```python
from build123d import *

# Parameters (mm, degrees)
SKETCH1_R           = 14
SKETCH1_R_2         = 12.425
BOSS_EXTRUDE1_DEPTH = 30
SKETCH2_W           = 40
SKETCH2_H           = 3
BOSS_EXTRUDE2_DEPTH = 30
SKETCH3_R           = 1.5
CUT_EXTRUDE1_DEPTH  = 30


with BuildPart() as part:
    # Sketch1 → Boss-Extrude1 (new body)
    with BuildSketch(Plane(origin=(0, 0, 0), x_dir=(1, 0, 0), z_dir=(0, 1, 0))):
        with Locations(Location((0, 0, 0), (0, 0, 270))):
            Circle(SKETCH1_R)
        with Locations(Location((0, 0, 0), (0, 0, 270))):
            Circle(SKETCH1_R_2, mode=Mode.SUBTRACT)
    extrude(amount=BOSS_EXTRUDE1_DEPTH)

    # Sketch2 → Boss-Extrude2 (add)
    with BuildSketch(Plane.XZ):
        with Locations((0, -14)):
            Rectangle(SKETCH2_W, SKETCH2_H)
    extrude(amount=-BOSS_EXTRUDE2_DEPTH)

    # Sketch3 → Cut-Extrude1 (cut)
    with BuildSketch(Plane.XY.offset(-12.5)):
        with Locations((17, 23)):
            Circle(SKETCH3_R)
        with Locations((-17, 23)):
            Circle(SKETCH3_R)
        with Locations((17, 7)):
            Circle(SKETCH3_R)
        with Locations((-17, 7)):
            Circle(SKETCH3_R)
    extrude(amount=-CUT_EXTRUDE1_DEPTH, mode=Mode.SUBTRACT)


solid = part.part
```
Work out the finished part from the listing and answer in its coordinate system (mm). A direction names the side the tool comes from. Coordinates: 2 decimals unless noted, no trailing zeros. Order: outer loops, then holes, each group sorted by start corner. A loop starts at its lowest first (then second) coordinate and runs counter-clockwise, first axis right, second up. Notation, with made-up numbers: (-27, -32) - (21, -32) arc R24 cw to (21, -13) - close; hole circle Ø2 at (64.5, 35). An arc over 180 degrees is marked (long way). Answer as a JSON object with one key per item and string values.
1. The mould has two halves that part along Y. Classify faces 4 (the face through (-18.5, 7.07, -13.98)), 5 (the face through (15.8, 6.1, -14)), 6 (the face through (-2, 30, -13)), 7 (the face through (-20, 15, -14)): +Y half, -Y half, draft (parallel to the pull), parting line (faces both ways), or undercut.
Output values:
{"face 4": "undercut", "face 5": "undercut", "face 6": "+Y half", "face 7": "draft"}
2. Find section B-B on z = 0. Determine the outline of the cut face in (x, y) (3 decimals), plus the area to 3 significant figures.
Output values:
{"outline": "(-14, 0) - (-12.425, 0) - (-12.425, 30) - (-14, 30) - close; (12.425, 0) - (14, 0) - (14, 30) - (12.425, 30) - close", "area": "94.5 mm²"}
3. Find section D-D on x = 0. Determine the outline of the cut face in (y, z) (3 decimals), plus the area to 4 significant figures.
Output values:
{"outline": "(0, -15.5) - (30, -15.5) - (30, -12.425) - (0, -12.425) - close; (0, 12.425) - (30, 12.425) - (30, 14) - (0, 14) - close", "area": "139.5 mm²"}
4. Consider line 1 (Y direction, x = 17, z = -13.2); line 2 (Z direction, x = 16, y = 27.75); line 3 (Z direction, x = -9.5, y = 15.25). Determine where each line is inside the solid, lowest interval first.
Output values:
{"line 1": "y = 0 to 5.5, 8.5 to 21.5, 24.5 to 30", "line 2": "z = -15.5 to -12.5", "line 3": "z = -15.5 to -12.5, -10.28 to -8.01, 8.01 to 10.28"}
5. Find section A-A on y = 7. Determine the outline of the cut face in (x, z) (3 decimals), plus the area to 3 significant figures.
Output values:
{"outline": "(-20, -15.5) - (-18.5, -15.5) - (-18.5, -12.5) - (-20, -12.5) - close; (-15.5, -15.5) - (15.5, -15.5) - (15.5, -12.5) - (6.305, -12.5) arc R14 ccw (long way) to (-6.305, -12.5) - (-15.5, -12.5) - close; (18.5, -15.5) - (20, -15.5) - (20, -12.5) - (18.5, -12.5) - close; hole circle Ø24.85 at (0, 0)", "area": "220 mm²"}
6. Each of these flat-tipped pins is pushed along its axis until it touches: P1, Ø12, axis at x = -0.5, z = 6.5, coming from the -Y side; P2, Ø15, axis at x = -14.5, y = 13, coming from the +Z side; P3, Ø15, axis at x = 14, y = 10.5, coming from the +Z side; P4, Ø3.5, axis at x = 17, y = 23, coming from the +Z side. Where does it stop, or does it pass through?
Output values:
{"P1": "stops at y = 0", "P2": "stops at z = 12.12", "P3": "stops at z = 12.4", "P4": "stops at z = -12.5"}
7. Find section C-C on x = -8. Determine the outline of the cut face in (y, z).
Output values:
{"outline": "(0, -15.5) - (30, -15.5) - (30, -12.5) - (0, -12.5) - close; (0, -11.49) - (30, -11.49) - (30, -9.51) - (0, -9.51) - close; (0, 9.51) - (30, 9.51) - (30, 11.49) - (0, 11.49) - close"}
8. A tool of negligible diameter and unlimited length cuts with its end or side. For faces 1 (the face through (13, 15, -12.5)), 2 (the face through (-13, 15, -12.5)), 3 (the face through (-2, 0, -13)), from which of +Z, -Z, +X, -X, +Y, -Y can it reach the whole face along a straight path? Write none if from no direction.
Output values:
{"face 1": "+X, +Y, -Y", "face 2": "-X, +Y, -Y", "face 3": "+Z, -Z, +X, -X, -Y"}
